Read the model definition and answer for the solid it produces. Units are mm, in the model's axes. Give positions to 0.01 mm unless a question says otherwise; leave off trailing zeros. Order: outer loops, then holes, each group sorted by start corner. A loop starts at its lowest first (then second) coordinate and runs counter-clockwise, first axis right, second up. Notation, with made-up numbers: (28.5, -6) - (53.5, -6) arc R19 cw to (53.5, 29) - close; hole circle Ø2 at (-7.5, 39). An arc over 180 degrees is marked (long way). Write item = value, one per line.
```python
from build123d import *

# Parameters (mm, degrees)
CROQUIS1_R              = 1.5
CROQUIS1_R_2            = 5
SALIENTE_EXTRUIR1_DEPTH = 3
CROQUIS2_R              = 1
CORTAR_EXTRUIR2_DEPTH   = 43.532340636


with BuildPart() as part:
    # Croquis1 → Saliente-Extruir1 (new body)
    with BuildSketch(Plane.XY):
        with BuildLine():
            ThreePointArc((-5.006412365, -24.493587635), (-4.990675805, -24.496798873), (-4.974937186, -24.5))
            ThreePointArc((-4.974937186, -24.5), (-0.250313875, -29.993730366), (5, -25))
            ThreePointArc((5, -25), (5.261221354, -21.77810342), (6.038061758, -18.640369658))
            ThreePointArc((6.038061758, -18.640369658), (8.90430573, -16.264636165), (9.334316304, -12.56672391))
            ThreePointArc((9.334316304, -12.56672391), (16.073984628, -7.10233955), (24.493587635, -5.006412365))
            ThreePointArc((24.493587635, -5.006412365), (24.496798873, -4.990675805), (24.5, -4.974937186))
            ThreePointArc((24.5, -4.974937186), (29.993730366, -0.250313875), (25, 5))
            ThreePointArc((25, 5), (21.77810342, 5.261221354), (18.640369658, 6.038061758))
            ThreePointArc((18.640369658, 6.038061758), (16.264636165, 8.90430573), (12.56672391, 9.334316304))
            ThreePointArc((12.56672391, 9.334316304), (7.10233955, 16.073984628), (5.006412365, 24.493587635))
            ThreePointArc((5.006412365, 24.493587635), (4.990675805, 24.496798873), (4.974937186, 24.5))
            ThreePointArc((4.974937186, 24.5), (0.250313875, 29.993730366), (-5, 25))
            ThreePointArc((-5, 25), (-5.261221354, 21.77810342), (-6.038061758, 18.640369658))
            ThreePointArc((-6.038061758, 18.640369658), (-8.90430573, 16.264636165), (-9.334316304, 12.56672391))
            ThreePointArc((-9.334316304, 12.56672391), (-16.073984628, 7.10233955), (-24.493587635, 5.006412365))
            ThreePointArc((-24.493587635, 5.006412365), (-24.496798873, 4.990675805), (-24.5, 4.974937186))
            ThreePointArc((-24.5, 4.974937186), (-29.993730366, 0.250313875), (-25, -5))
            ThreePointArc((-25, -5), (-21.77810342, -5.261221354), (-18.640369658, -6.038061758))
            ThreePointArc((-18.640369658, -6.038061758), (-16.264636165, -8.90430573), (-12.56672391, -9.334316304))
            ThreePointArc((-12.56672391, -9.334316304), (-7.10233955, -16.073984628), (-5.006412365, -24.493587635))
        make_face()
        with Locations((-25, 0)):
            Circle(CROQUIS1_R, mode=Mode.SUBTRACT)
        with Locations((0, -25)):
            Circle(CROQUIS1_R, mode=Mode.SUBTRACT)
        with Locations((4.50977544, -13.879661629)):
            Circle(CROQUIS1_R, mode=Mode.SUBTRACT)
        with Locations((0, 25)):
            Circle(CROQUIS1_R, mode=Mode.SUBTRACT)
        with Locations((13.879661629, 4.50977544)):
            Circle(CROQUIS1_R, mode=Mode.SUBTRACT)
        with Locations((25, 0)):
            Circle(CROQUIS1_R, mode=Mode.SUBTRACT)
        with Locations((-4.50977544, 13.879661629)):
            Circle(CROQUIS1_R, mode=Mode.SUBTRACT)
        with Locations((-13.879661629, -4.50977544)):
            Circle(CROQUIS1_R, mode=Mode.SUBTRACT)
        Circle(CROQUIS1_R_2, mode=Mode.SUBTRACT)
    extrude(amount=SALIENTE_EXTRUIR1_DEPTH)

    # Croquis2 → Cortar-Extruir2 (cut, through all)
    with BuildSketch(Plane.XY.offset(3)):
        with Locations((3.75, 6.495190528)):
            Circle(CROQUIS2_R)
        with Locations((3.75, -6.495190528)):
            Circle(CROQUIS2_R)
        with Locations((-7.5, 0)):
            Circle(CROQUIS2_R)
    extrude(amount=-CORTAR_EXTRUIR2_DEPTH, mode=Mode.SUBTRACT)


solid = part.part
```
1. Straight lines are drawn through the part: L1, parallel to Y at x = 0, z = 0.7; L2, parallel to Y at x = -25, z = 1.1; L3, parallel to X at y = 4.5, z = 0.65. For each, find the intervals that lie inside material, in ascending order. Write a range as [from, to].
Recorded:
L1 = [-30, -26.5], [-23.5, -5], [5, 23.5], [26.5, 30]
L2 = [-5, -1.5], [1.5, 5]
L3 = [-27.18, -2.18], [2.18, 12.38], [15.38, 27.18]
2. Section A-A (x = 0) is taken. Determine the outline of the cut face in (y, z).
Recorded:
outline = (-30, 0) - (-26.5, 0) - (-26.5, 3) - (-30, 3) - close; (-23.5, 0) - (-5, 0) - (-5, 3) - (-23.5, 3) - close; (5, 0) - (23.5, 0) - (23.5, 3) - (5, 3) - close; (26.5, 0) - (30, 0) - (30, 3) - (26.5, 3) - close
3. Determine the mould class of faces 1 (the face through (-2, 5, 0)), 2 (the face through (5.254, -21.823, 1.479)), 3 (the face through (-12.5, -5.1, 1.5)) for opening direction X: +X half, -X half, draft (parallel to the pull), parting line (faces both ways), or undercut.
Recorded:
face_1 = draft
face_2 = +X half
face_3 = undercut
4. Flat-ended cylindrical pins translate along their axes: pin 1 (1.5 mm diameter, centred on y = 12, z = 0.5, fed in from +X); pin 2 (1 mm diameter, centred on y = -18, z = 2, fed in from +X). Find the tip coordinate at first contact, or state that the pin passes through.
Recorded:
pin_1 = 10.48
pin_2 = 7.96
5. Section C-C (x = 11.5) is taken. Determine the outline of the cut face in (y, z).
Recorded:
outline = (-10.24, 0) - (10.24, 0) - (10.24, 3) - (-10.24, 3) - close
6. Section B-B (z = 2.35) is taken. Count the separate pieces of the cut face and the enclosed holes in it, and give its area (3 significant figures).
Recorded:
separate_pieces = 1
enclosed_holes = 12
area = 1,290 mm^2
